Design review of the part built by this model. Coordinates are the model's own, in mm. Coordinates: 2 decimals unless noted, no trailing zeros. Loops run counter-clockwise (first coordinate to the right, second up) from the corner with the lowest first, then second, coordinate; pieces in that order, holes last. Notation, with made-up numbers: (-28, 65) - (-9, 65) arc R25 cw to (-9, 92) - close; hole circle Ø6 at (29, -17.75). An arc over 180 degrees is marked (long way). Return JSON: item names as keys, results as strings. Group by question number.
from build123d import *

# Parameters (mm, degrees)
F0_R     = 0.155
F1_DEPTH = 20
F2_R     = 0.155
F3_ANGLE = 270
F4_R     = 0.155
F5_DEPTH = 0.15


with BuildPart() as f1:
    # F0 (on Top) → F1 (new body)
    with BuildSketch(Plane.XY):
        Circle(F0_R)
    extrude(amount=F1_DEPTH)

    # F2 (on face) → F3 (revolve)
    with BuildSketch(Plane.XY.offset(20)):
        Circle(F2_R)
    revolve(axis=Axis((0.0432368064, 0.718167399, 20), (-1, 0, 0)), revolution_arc=F3_ANGLE)

    # F4 (on face) → F5 (join)
    with BuildSketch(Plane.XZ.offset(-0.718167399)):
        with Locations((0, 19.281832601)):
            Circle(F4_R)
    extrude(amount=F5_DEPTH)


solid = f1.part
Item 1: To check wall thickness, follow line 1 (Z direction, x = -0.1, y = 0.85); line 2 (Z direction, x = 0.05, y = 1.2); line 3 (Y direction, x = 0, z = 19.25) (3 decimals). State the ranges of each line that lie inside material, in increasing order. Write a range as from..to.
Item 2: Add section A-A (x = 0). State the section outline as (y, z) points (3 decimals), then the cut area to 3 significant figures.
Item 3: Add section B-B (z = 3.25). State the section outline as (x, y) points (3 decimals).
Answers below:
{
 "1": {"line 1": "z = 19.17..19.41, 20.59..20.83", "line 2": "z = 19.28..19.69, 20.31..20.72", "line 3": "y = -0.155..0.155, 0.568..1.165"},
 "2": {"outline": "(-0.155, 0) - (0.155, 0) - (0.155, 20) arc R0.563 cw (long way) to (0.718, 19.437) - (0.568, 19.437) - (0.568, 19.127) - (0.718, 19.127) arc R0.873 ccw (long way) to (-0.155, 20) - close", "area": "7.30 mm^2"},
 "3": {"outline": "circle Ø0.31 at (0, 0)"}
}
